from build123d import *

# Parameters (mm, degrees)
SKETCH1_R               = 2.25
SKETCH1_R_2             = 1.65
BOSS_EXTRUDE1_DEPTH     = 6
CUT_EXTRUDE1_DEPTH      = 1
CUT_EXTRUDE1_DEPTH_BACK = 7
SKETCH3_R               = 3.5
BOSS_EXTRUDE2_DEPTH     = 7.1
CHAMFER1_SIZE           = 2
BOSS_EXTRUDE3_DEPTH     = 6
FILLET1_R               = 10


with BuildPart() as part:
    # Sketch1 → Boss-Extrude1 (new body)
    with BuildSketch(Plane(origin=(0, 0, 0), x_dir=(1, 0, 0), z_dir=(0, 1, 0))):
        Polygon((0, 0), (108, 0), (108, 6), (79, 16), (79, 96), (29, 96), (29, 16), (0, 6), align=None)
        with Locations((4, 3)):
            Circle(SKETCH1_R, mode=Mode.SUBTRACT)
        with Locations((104, 3)):
            Circle(SKETCH1_R, mode=Mode.SUBTRACT)
        with Locations((39, 91)):
            Circle(SKETCH1_R_2, mode=Mode.SUBTRACT)
        with Locations((69, 91)):
            Circle(SKETCH1_R_2, mode=Mode.SUBTRACT)
        with Locations((39, 21)):
            Circle(SKETCH1_R_2, mode=Mode.SUBTRACT)
        with Locations((69, 21)):
            Circle(SKETCH1_R_2, mode=Mode.SUBTRACT)
    extrude(amount=BOSS_EXTRUDE1_DEPTH)

    # Sketch2 → Cut-Extrude1 (cut, two sides)
    with BuildSketch(Plane(origin=(0, 6, 0), x_dir=(1, 0, 0), z_dir=(0, 1, 0))) as cut_extrude1_sk:
        with BuildLine():
            Line((19, 0), (89, 0))
            ThreePointArc((89, 0), (54, 5.217597168), (19, 0))
        make_face()
    extrude(amount=CUT_EXTRUDE1_DEPTH, mode=Mode.SUBTRACT)
    extrude(cut_extrude1_sk.sketch, amount=-CUT_EXTRUDE1_DEPTH_BACK, mode=Mode.SUBTRACT)

    # Sketch3 → Boss-Extrude2 (add)
    with BuildSketch(Plane.XZ):
        with Locations((36.5, -81)):
            Circle(SKETCH3_R)
        with Locations((71.5, -81)):
            Circle(SKETCH3_R)
    extrude(amount=BOSS_EXTRUDE2_DEPTH)

    # Chamfer1
    chamfer1_edges = [part.edges().sort_by_distance(p)[0] for p in [
        (33, 0, -81),
        (68, 0, -81),
    ]]
    chamfer(chamfer1_edges, length=CHAMFER1_SIZE)

    # Sketch4 → Boss-Extrude3 (add)
    with BuildSketch(Plane(origin=(0, 6, 0), x_dir=(1, 0, 0), z_dir=(0, 1, 0))):
        with BuildLine():
            Line((0, 0), (0, -1))
            Line((0, -1), (15.874355013, -1))
            ThreePointArc((15.874355013, -1), (17.433758893, -0.489314628), (19, 0))
            Line((19, 0), (0, 0))
        make_face()
        with BuildLine():
            Line((108, -1), (92.125644987, -1))
            ThreePointArc((92.125644987, -1), (90.566241107, -0.489314628), (89, 0))
            Line((89, 0), (108, 0))
            Line((108, 0), (108, -1))
        make_face()
    extrude(amount=-BOSS_EXTRUDE3_DEPTH)

    # Fillet1
    fillet1_edges = [part.edges().sort_by_distance(p)[0] for p in [
        (29, 3, -16),
        (29, 3, -96),
        (79, 3, -96),
        (79, 3, -16),
        (15.874355013, 3, 1),
        (92.125644987, 3, 1),
    ]]
    fillet(fillet1_edges, radius=FILLET1_R)


solid = part.part
Geometry: final body of the model. Coordinates: model frame, mm. A direction names the side the tool comes from. Give positions to 0.01 mm unless a question says otherwise; leave off trailing zeros. Write each loop counter-clockwise with the first axis right and the second up, starting at its lowest first coordinate (ties: lowest second). Pieces come first, ordered by that corner, then holes.
(1) First-contact query: P1, Ø6.5, axis at y = 2.5, z = -47.5, coming from the -X side; P2, Ø4, axis at x = 39, z = -91, coming from the -Y side; P3, Ø6, axis at x = 37.5, y = 1, coming from the +Z side; P4, Ø2.5, axis at x = 69, z = -21, coming from the -Y side. Flat tips, straight axial feed; report the tip coordinate or a pass-through.
(2) Cut plane B-B, the plane z = -3. Return loops of the section in (x, y).
(3) Cut plane C-C, the plane y = -4. Return loops of the section in (x, z), then the cut area to 3 significant figures.
(4) Cut plane A-A, the plane y = 1.75. Return loops of the section in (x, z).
(5) Access query for faces 4 (the flat face through (29, 3, -55)), 5 (the cylindrical face through (92.198, 2.958, 0.883)), 6 (the cylindrical face through (35.741, -4.514, -84.417)), 7 (the cylindrical face through (6.08, 2.96, -2.14)). Directions: +Z, -Z, +X, -X, +Y, -Y. A direction counts if a zero-diameter tool reaches every point of the face in a straight line with its end or side. Return the directions, or none.
(6) Mould query, pull axis Z, two halves, no side actions, for faces 1 (the cylindrical face through (37.35, 2.96, -21.07)), 2 (the cylindrical face through (15.845, 2.958, 0.876)), 3 (the flat face through (79, 3, -54)). Classes: released by +Z, released by -Z, zero draft, split by the parting line, or undercut.
(7) Ray query, line 1 (X direction, y = 3.75, z = -21); line 2 (X direction, y = 4.5, z = -91); line 3 (Z direction, x = 69, y = 3.6). Return the intervals inside material, ascending.
(8) Cut plane D-D, the plane x = 4. Return loops of the section in (y, z).
Values follow:
1. P1: stops at x = 29
1. P2: stops at y = 0
1. P3: stops at z = -3.62
1. P4: passes through
2. outline: (0, 0) - (1.75, 0) - (1.75, 6) - (0, 6) - close; (6.25, 0) - (31.04, 0) - (31.04, 6) - (6.25, 6) - close; (76.96, 0) - (101.75, 0) - (101.75, 6) - (76.96, 6) - close; (106.25, 0) - (108, 0) - (108, 6) - (106.25, 6) - close
3. outline: circle Ø7 at (36.5, -81); circle Ø7 at (71.5, -81)
3. area: 77.0 mm2
4. outline: (0, -6) - (22.26, -13.68) arc R10 cw to (29, -23.13) - (29, -86) arc R10 ccw to (39, -96) - (69, -96) arc R10 ccw to (79, -86) - (79, -23.13) arc R10 cw to (85.74, -13.68) - (108, -6) - (108, 1) - (93.72, 1) arc R10 ccw to (90.67, 0.52) arc R120 cw to (17.33, 0.52) arc R10 ccw to (14.28, 1) - (0, 1) - close; hole circle Ø4.5 at (4, -3); hole circle Ø3.3 at (39, -91); hole circle Ø3.3 at (39, -21); hole circle Ø3.3 at (69, -91); hole circle Ø3.3 at (69, -21); hole circle Ø4.5 at (104, -3)
5. face 4: -Z, -X, +Y, -Y
5. face 5: +Z, +Y, -Y
5. face 6: -Y
5. face 7: +Y, -Y
6. face 1: undercut
6. face 2: released by +Z
6. face 3: zero draft
7. line 1: x = 28.77 to 37.35, 40.65 to 67.35, 70.65 to 79.23
7. line 2: x = 30.34 to 37.35, 40.65 to 67.35, 70.65 to 77.66
7. line 3: z = -96 to -92.65, -89.35 to -22.65, -19.35 to -4.28
8. outline: (0, -7.38) - (6, -7.38) - (6, -5.25) - (0, -5.25) - close; (0, -0.75) - (6, -0.75) - (6, 1) - (0, 1) - close
